Part print with two shaded views. Sizes in mm from the minimum x, y, z corner. Give positions to 0.01 mm unless a question says otherwise; leave off trailing zeros. Order: outer loops, then holes, each group sorted by start corner. A loop starts at its lowest first (then second) coordinate and runs counter-clockwise, first axis right, second up. Notation, with made-up numbers: M -38,-9 L -18,-9 A6 cw -18,-2 Z; hole C 68,82.5 d7. An arc over 180 degrees is marked long. Answer as CSV lines item,"result".
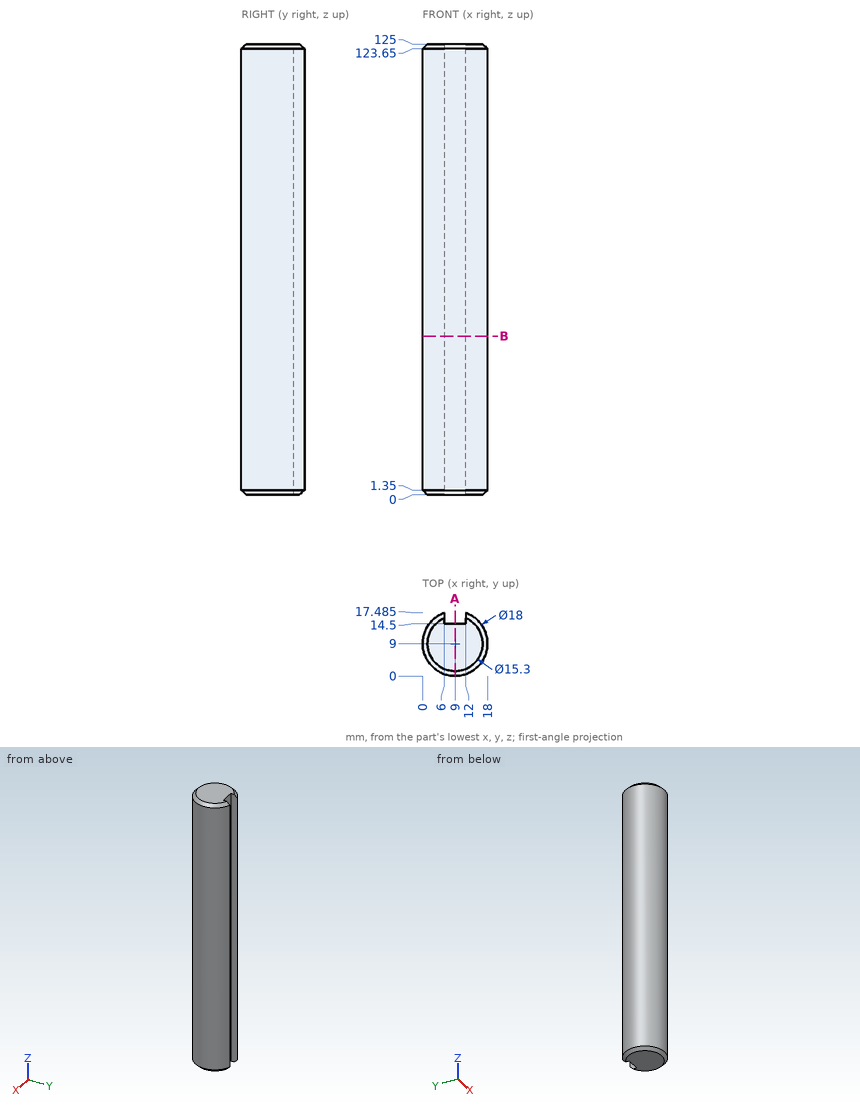
Item 1: Band-saw the part on B-B (z = 44). Give the cut face in (x, y) (1 decimal), and give its area (4 significant figures).
Geometry says:
outline,"M 6,14.5 L 6,17.5 A9 ccw long 12,17.5 L 12,14.5 Z"
area,"234.5 mm2"
Item 2: Probe line 1 along Y through (x, z) = (9.25, 89); line 2 along X through (y, z) = (8.5, 103.5); line 3 along Y through (x, z) = (13.75, 19) (1 decimal). List the from-to ranges inside material, lowest first. Write a range as from..to.
Geometry says:
line 1,"y = 0..14.5"
line 2,"x = 0.01..17.99"
line 3,"y = 1.4..16.6"
Item 3: Band-saw the part on A-A (x = 9). Give the cut face in (y, z), and give its area (3 significant figures).
Geometry says:
outline,"M 0,1.35 L 1.35,0 L 14.5,0 L 14.5,125 L 1.35,125 L 0,123.65 Z"
area,"1,810 mm2"
Item 4: Drop flat-ended pins along their axis: pin 1 (6 mm diameter, centred on x = 9.5, z = 94, fed in from +Y) (1 decimal); pin 2 (2 mm diameter, centred on y = 4, z = 61, fed in from -X); pin 3 (1.5 mm diameter, centred on y = 16.5, z = 83.5, fed in from +X). Give the stop position or say it passes through.
Geometry says:
pin 1,"stops at y = 17.5"
pin 2,"stops at x = 0.94"
pin 3,"stops at x = 14.95"
